from build123d import *

# Parameters (mm, degrees)
PAD_DEPTH       = 20
SKETCH001_W     = 23.8
SKETCH001_H     = 46
POCKET_DEPTH    = 18
SKETCH002_R     = 8.2
POCKET001_DEPTH = 5
SKETCH003_R     = 1.7
POCKET002_DEPTH = 5
SKETCH004_R     = 1.7
POCKET003_DEPTH = 5
SKETCH005_W     = 25.8
SKETCH005_H     = 2
SKETCH005_W_2   = 2
SKETCH005_H_2   = 48
SKETCH005_W_3   = 23.8
SKETCH005_H_3   = 50
PAD001_DEPTH    = 15
SKETCH006_W     = 23.8
SKETCH006_H     = 46
POCKET004_DEPTH = 15


with BuildPart() as part:
    # Sketch → Pad (new body)
    with BuildSketch(Plane.XY):
        Polygon((-2, 15.090214), (0, 15.090214), (0, -54.909786), (-2, -54.909786), (-2, -44.909786), (-27.8, -44.909786), (-27.8, 5.090214), (-2, 5.090214), align=None)
    extrude(amount=PAD_DEPTH)

    # Sketch001 (on Face9 of Pad) → Pocket (cut)
    with BuildSketch(Plane(origin=(0, 0, 0), x_dir=(1, 0, 0), z_dir=(0, 0, -1))):
        with Locations((-13.9, 19.909786)):
            Rectangle(SKETCH001_W, SKETCH001_H)
    extrude(amount=-POCKET_DEPTH, mode=Mode.SUBTRACT)

    # Sketch002 (on Face5 of Pocket) → Pocket001 (cut)
    with BuildSketch(Plane.XY.offset(20)):
        with Locations((-13.5, -9.004213)):
            Circle(SKETCH002_R)
        with Locations((-13.5, -31.004213)):
            Circle(SKETCH002_R)
    extrude(amount=-POCKET001_DEPTH, mode=Mode.SUBTRACT)

    # Sketch003 (on Face9 of Pocket001) → Pocket002 (cut)
    with BuildSketch(Plane(origin=(-2, 0, 0), x_dir=(0, -1, 0), z_dir=(-1, 0, 0))):
        with Locations((49.909786, 10)):
            Circle(SKETCH003_R)
    extrude(amount=-POCKET002_DEPTH, mode=Mode.SUBTRACT)

    # Sketch004 (on Face2 of Pocket002) → Pocket003 (cut)
    with BuildSketch(Plane(origin=(-2, 0, 0), x_dir=(0, -1, 0), z_dir=(-1, 0, 0))):
        with Locations((-10.090214, 10)):
            Circle(SKETCH004_R)
    extrude(amount=-POCKET003_DEPTH, mode=Mode.SUBTRACT)

    # Sketch005 (on Face4 of Pocket003) → Pad001 (join)
    with BuildSketch(Plane(origin=(0, 0, 0), x_dir=(1, 0, 0), z_dir=(0, 0, -1))):
        with Locations((-14.9, 43.909786)):
            Rectangle(SKETCH005_W, SKETCH005_H)
        with Locations((-26.8, 18.909786)):
            Rectangle(SKETCH005_W_2, SKETCH005_H_2)
        with Locations((-13.9, -4.090214)):
            Rectangle(SKETCH005_W_3, SKETCH005_H)
        with Locations((-1, 19.909786)):
            Rectangle(SKETCH005_W_2, SKETCH005_H_3)
    extrude(amount=PAD001_DEPTH)

    # Sketch006 (on Face21 of Pad001) → Pocket004 (cut)
    with BuildSketch(Plane(origin=(0, 0, -15), x_dir=(1, 0, 0), z_dir=(0, 0, -1))):
        with Locations((-13.9, 19.909786)):
            Rectangle(SKETCH006_W, SKETCH006_H)
    extrude(amount=-POCKET004_DEPTH, mode=Mode.SUBTRACT)


solid = part.part
Design review of the part built by this model. Coordinates are the model's own, in mm. A direction names the side the tool comes from. Round coordinates to 2 decimals unless told otherwise and drop trailing zeros. Write each loop counter-clockwise with the first axis right and the second up, starting at its lowest first coordinate (ties: lowest second). Pieces come first, ordered by that corner, then holes. Notation, with made-up numbers: (-39, 60) - (-25, 60) arc R26 cw to (-25, 89) - close; hole circle Ø1 at (9.5, 45). An arc over 180 degrees is marked (long way). Use a Markdown table: item, result. Add a question column.
1. We need section C-C (y = -15). State the section outline as (x, z) points.
2. We need section D-D (z = 16). State the section outline as (x, y) points.
3. For faces 5 (the face through (-1, 10, 0)), 6 (the face through (-14, -20, 18)), 7 (the face through (-2, 12, 10)), 8 (the face through (-2, -52, 10)), list the 3-axis set-ups (+Z, -Z, +X, -X, +Y, -Y) from which the entire face can be reached by the end or side of a thin tool; tool diameter is ignored.
4. Clearance check with flat-ended pins moving along their axes: pin 1 (0.6 mm diameter, centred on x = -0.5, y = 11, fed in from -Z); pin 2 (11 mm diameter, centred on y = -48, z = 6, fed in from -X); pin 3 (15 mm diameter, centred on x = -13.5, y = -9, fed in from +Z); pin 4 (1.5 mm diameter, centred on x = -11, z = 8.5, fed in from -Y). State where each tip first meets the part, or that it passes through.
5. Mouldability with a two-part tool opening along X and no side actions: class faces 1 (the face through (-25.8, -20, 2)), 2 (the face through (-27.8, -20, 3)), 3 (the face through (-1, -54.91, 10)), 4 (the face through (-2, -20, 2)) as +X half, -X half, draft (parallel to the pull), parting line (faces both ways), or undercut.
6. Wall thickness on probe 1 along Y at (x, z) = (-13.5, 19.5); probe 2 along X at (y, z) = (-37.5, 14); probe 3 along Y at (x, z) = (-9.75, -1): over which ranges is each line inside the solid? List them lowest first.
7. We need section B-B (x = -13.5). State the section outline as (y, z) points.
8. We need section A-A (z = 9). State the section outline as (x, y) points.
Output:
| question | item | result |
|---|---|---|
| 1 | outline | (-27.8, -15) - (-25.8, -15) - (-25.8, 18) - (-19.09, 18) - (-19.09, 20) - (-27.8, 20) - close; (-7.91, 18) - (-2, 18) - (-2, -15) - (0, -15) - (0, 20) - (-7.91, 20) - close |
| 2 | outline | (-27.8, -44.91) - (-2, -44.91) - (-2, -54.91) - (0, -54.91) - (0, 15.09) - (-2, 15.09) - (-2, 5.09) - (-27.8, 5.09) - close; hole (-25.8, -42.91) - (-2, -42.91) - (-2, 3.09) - (-25.8, 3.09) - close |
| 3 | face 5 | -Z, +X, -X, +Y |
| 3 | face 6 | -Z |
| 3 | face 7 | +Z, -Z, -X, +Y |
| 3 | face 8 | +Z, -Z, -X, -Y |
| 4 | pin 1 | stops at z = 0 |
| 4 | pin 2 | stops at x = -27.8 |
| 4 | pin 3 | passes through |
| 4 | pin 4 | stops at y = -44.91 |
| 5 | face 1 | undercut |
| 5 | face 2 | -X half |
| 5 | face 3 | draft |
| 5 | face 4 | undercut |
| 6 | probe 1 | y = -44.91 to -39.2, -22.8 to -17.2, -0.8 to 5.09 |
| 6 | probe 2 | x = -27.8 to -25.8, -2 to 0 |
| 6 | probe 3 | y = -44.91 to -42.91, 3.09 to 5.09 |
| 7 | outline | (-44.91, -15) - (-42.91, -15) - (-42.91, 18) - (-39.2, 18) - (-39.2, 20) - (-44.91, 20) - close; (-22.8, 18) - (-17.2, 18) - (-17.2, 20) - (-22.8, 20) - close; (-0.8, 18) - (3.09, 18) - (3.09, -15) - (5.09, -15) - (5.09, 20) - (-0.8, 20) - close |
| 8 | outline | (-27.8, -44.91) - (-2, -44.91) - (-2, -48.54) - (0, -48.54) - (0, 8.72) - (-2, 8.72) - (-2, 5.09) - (-27.8, 5.09) - close; (-2, -54.91) - (0, -54.91) - (0, -51.28) - (-2, -51.28) - close; (-2, 11.46) - (0, 11.46) - (0, 15.09) - (-2, 15.09) - close; hole (-25.8, -42.91) - (-2, -42.91) - (-2, 3.09) - (-25.8, 3.09) - close |
